```python
from build123d import *

# Parameters (mm, degrees)
SKETCH_W               = 20
SKETCH_H               = 30
PAD_DEPTH              = 3
SKETCH001_W            = 2
SKETCH001_H            = 29.849984
PAD001_DEPTH           = 150
PAD002_DEPTH           = 150
POCKET_DEPTH           = 8
POCKET001_DEPTH        = 2.25
POCKET002_DEPTH        = 2.25
SKETCH008_W            = 10
SKETCH008_H            = 5
POCKET003_DEPTH        = 2.5
SKETCH009_W            = 10
SKETCH009_H            = 10
POCKET004_DEPTH        = 5
SKETCH010_W            = 1
SKETCH010_H            = 150.25
POCKET005_DEPTH        = 1
SKETCH011_W            = 5
SKETCH011_H            = 0.5
POCKET006_DEPTH        = 1
LINEARPATTERN_COUNT    = 16
LINEARPATTERN_PITCH    = 10
SKETCH012_W            = 2.5
SKETCH012_H            = 0.5
POCKET007_DEPTH        = 1
LINEARPATTERN001_COUNT = 15
LINEARPATTERN001_PITCH = 10
SKETCH013_R            = 0.5
POCKET008_DEPTH        = 5
LINEARPATTERN002_COUNT = 15
LINEARPATTERN002_PITCH = 10
SKETCH014_R            = 0.5
POCKET009_DEPTH        = 5
LINEARPATTERN003_COUNT = 14
LINEARPATTERN003_PITCH = 10


with BuildPart() as part:
    # Sketch → Pad (new body)
    with BuildSketch(Plane.XY):
        Rectangle(SKETCH_W, SKETCH_H)
    extrude(amount=PAD_DEPTH)

    # Sketch001 (on Face6 of Pad) → Pad001 (join)
    with BuildSketch(Plane.XY.offset(3)):
        with Locations((-9, 0)):
            Rectangle(SKETCH001_W, SKETCH001_H)
    extrude(amount=PAD001_DEPTH)

    # Sketch003 (on Face5 of Pad001) → Pad002 (join)
    with BuildSketch(Plane.XY.offset(3)):
        Polygon((-8.02879, 4), (9.97121, 4), (9.97121, -4), (-8.007794, -4), align=None)
    extrude(amount=PAD002_DEPTH)

    # Sketch005 (on Face10 of Pad002) → Pocket (cut)
    with BuildSketch(Plane.XZ.offset(4)):
        Polygon((-8, 153), (10, 153), (10, 3), align=None)
    extrude(amount=-POCKET_DEPTH, mode=Mode.SUBTRACT)

    # Sketch006 (on Face10 of Pocket) → Pocket001 (cut)
    with BuildSketch(Plane.XZ.offset(4)):
        Polygon((-5, 140), (-5, 6), (15, 6), align=None)
    extrude(amount=-POCKET001_DEPTH, mode=Mode.SUBTRACT)

    # Sketch007 (on Face12 of Pocket001) → Pocket002 (cut)
    with BuildSketch(Plane(origin=(0, 4, 0), x_dir=(-1, 0, 0), z_dir=(0, 1, 0))):
        Polygon((-13, 6), (5, 6), (5, 150), align=None)
    extrude(amount=-POCKET002_DEPTH, mode=Mode.SUBTRACT)

    # Sketch008 (on Face5 of Pocket002) → Pocket003 (cut)
    with BuildSketch(Plane.XY.offset(3)):
        Rectangle(SKETCH008_W, SKETCH008_H)
    extrude(amount=-POCKET003_DEPTH, mode=Mode.SUBTRACT)

    # Sketch009 (on Face5 of Pocket003) → Pocket004 (cut)
    with BuildSketch(Plane.XY.offset(3)):
        Rectangle(SKETCH009_W, SKETCH009_H)
    extrude(amount=POCKET004_DEPTH, mode=Mode.SUBTRACT)

    # Sketch010 (on Face3 of Pocket004) → Pocket005 (cut)
    with BuildSketch(Plane(origin=(-10, 0, 0), x_dir=(0, -1, 0), z_dir=(-1, 0, 0))):
        with Locations((-9.5, 75.125)):
            Rectangle(SKETCH010_W, SKETCH010_H)
    extrude(amount=-POCKET005_DEPTH, mode=Mode.SUBTRACT)

    # Sketch011 (on Face8 of Pocket005) → Pocket006 (cut)
    with BuildSketch(Plane(origin=(-10, 0, 0), x_dir=(0, -1, 0), z_dir=(-1, 0, 0))):
        with Locations((-7, 0)):
            Rectangle(SKETCH011_W, SKETCH011_H)
    pocket006 = extrude(amount=-POCKET006_DEPTH, mode=Mode.SUBTRACT)

    # LinearPattern: Pocket006 ×16
    with Locations(*[(0, 0, i * LINEARPATTERN_PITCH) for i in range(1, LINEARPATTERN_COUNT)]):
        add(pocket006, mode=Mode.SUBTRACT)

    # Sketch012 (on Face8 of LinearPattern) → Pocket007 (cut)
    with BuildSketch(Plane(origin=(-10, 0, 0), x_dir=(0, -1, 0), z_dir=(-1, 0, 0))):
        with Locations((-8.25, 5)):
            Rectangle(SKETCH012_W, SKETCH012_H)
    pocket007 = extrude(amount=-POCKET007_DEPTH, mode=Mode.SUBTRACT)

    # LinearPattern001: Pocket007 ×15
    with Locations(*[(0, 0, i * LINEARPATTERN001_PITCH) for i in range(1, LINEARPATTERN001_COUNT)]):
        add(pocket007, mode=Mode.SUBTRACT)

    # Sketch013 (on Face8 of LinearPattern001) → Pocket008 (cut)
    with BuildSketch(Plane(origin=(-10, 0, 0), x_dir=(0, -1, 0), z_dir=(-1, 0, 0))):
        with Locations((10, 10)):
            Circle(SKETCH013_R)
    pocket008 = extrude(amount=-POCKET008_DEPTH, mode=Mode.SUBTRACT)

    # LinearPattern002: Pocket008 ×15
    with Locations(*[(0, 0, i * LINEARPATTERN002_PITCH) for i in range(1, LINEARPATTERN002_COUNT)]):
        add(pocket008, mode=Mode.SUBTRACT)

    # Sketch014 (on Face8 of LinearPattern002) → Pocket009 (cut)
    with BuildSketch(Plane(origin=(-10, 0, 0), x_dir=(0, -1, 0), z_dir=(-1, 0, 0))):
        with Locations((6, 15)):
            Circle(SKETCH014_R)
    pocket009 = extrude(amount=-POCKET009_DEPTH, mode=Mode.SUBTRACT)

    # LinearPattern003: Pocket009 ×14
    with Locations(*[(0, 0, i * LINEARPATTERN003_PITCH) for i in range(1, LINEARPATTERN003_COUNT)]):
        add(pocket009, mode=Mode.SUBTRACT)


solid = part.part
```
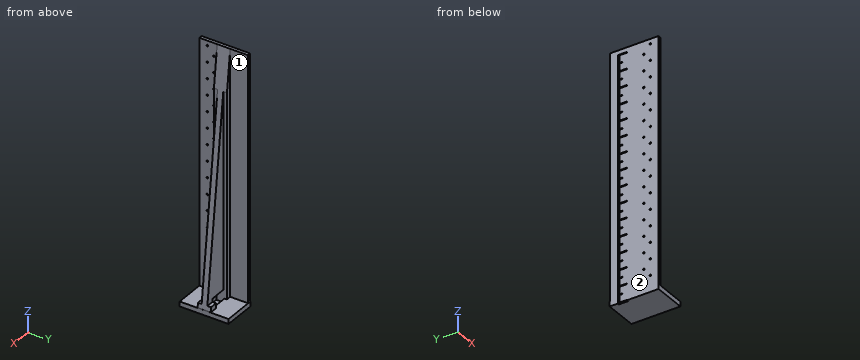
Can you work these out from the model? Positions are in its coordinate system, mm. Face numbers are marked on the shaded views. A direction names the side the tool comes from. Coordinates: 2 decimals unless noted, no trailing zeros. Loops run counter-clockwise (first coordinate to the right, second up) from the corner with the lowest first, then second, coordinate; pieces in that order, holes last.
1) I need wall thicknesses on probe 1 along Y at (x, z) = (-9.45, 40) (3 decimals); probe 2 along Y at (x, z) = (-9.55, 95) (3 decimals); probe 3 along Y at (x, z) = (-8.6, 110) (3 decimals). Which ranges of each line are inside material? Lowest first, please.
2) For pin 1 (2 mm diameter, centred on x = -9, z = 81, fed in from -Y) (3 decimals); pin 2 (0.6 mm diameter, centred on x = -9.5, z = 70, fed in from +Y) (3 decimals); pin 3 (1 mm diameter, centred on x = -4, z = 94, fed in from +Y); pin 4 (4 mm diameter, centred on x = -3, y = -2, fed in from -Z), each with a flat end and sliding along its axis, tell me the tip position at first contact or that it passes through.
3) Which directions (+Z, -Z, +X, -X, +Y, -Y) give clear straight access to the entire face, cutting with the end or side of a thin tool? Please do the marked faces 1 and 2.
4) Imagine slicing it at A-A on x = -0.5. List the corners of the cut face in (y, z) for me.
Completed:
1. probe 1: y = -14.925 to -10.5, -9.5 to 4.5, 10 to 14.925
1. probe 2: y = -14.925 to -6.5, -5.5 to 7, 10 to 14.925
1. probe 3: y = -14.925 to -10.5, -9.5 to 14.925
2. pin 1: stops at y = -14.925
2. pin 2: stops at y = 14.925
2. pin 3: stops at y = 1.75
2. pin 4: stops at z = 0
3. face 1: +Z, +X, +Y
3. face 2: +Z, -Z, -X, +Y, -Y
4. outline: (-15, 0) - (15, 0) - (15, 3) - (2.5, 3) - (2.5, 0.5) - (-2.5, 0.5) - (-2.5, 3) - (-15, 3) - close; (-1.75, 8) - (1.75, 8) - (1.75, 90.5) - (-1.75, 90.5) - close
